```python
from build123d import *

# Parameters (mm, degrees)
ESQUISSE2_R          = 3.5
BOSS_EXTRU_1_DEPTH   = 3.5
D_GAGEMENT_M31_D     = 3.4
D_GAGEMENT_M31_DEPTH = 3.5


with BuildPart() as part:
    # Esquisse1 → Révolution1 (revolve)
    with BuildSketch(Plane.XY, mode=Mode.PRIVATE) as r_volution1_sk:
        Polygon((0, 0), (-9.5, 0), (-9.5, 3.5), (-7.5, 3.5), (-6.95, 6), (-16.95, 6), (-16.95, 26), (-2.5, 26), (-2.5, 42), (0, 42), align=None)
    revolve(r_volution1_sk.sketch.rotate(Axis((0, 0, 0), (0, 1, 0)), 270), axis=Axis((0, 0, 0), (0, 1, 0)))

    # Esquisse2 → Boss.-Extru.1 (add)
    with BuildSketch(Plane(origin=(0, 0, 0), x_dir=(-1, 0, 0), z_dir=(0, -1, 0))):
        with Locations((6.717514421, -6.717514421)):
            Circle(ESQUISSE2_R)
        with Locations((-6.717514421, -6.717514421)):
            Circle(ESQUISSE2_R)
        with Locations((-6.717514421, 6.717514421)):
            Circle(ESQUISSE2_R)
        with Locations((6.717514421, 6.717514421)):
            Circle(ESQUISSE2_R)
    extrude(amount=-BOSS_EXTRU_1_DEPTH)

    # Dégagement M31
    with Locations(Plane(origin=(-6.717514421, 0, 6.717514421), x_dir=(0, 0, -1), z_dir=(0, -1, 0))):
        with Locations((0, 0), (0, 13.435028842), (13.435028842, 13.435028842), (13.435028842, 0)):
            Hole(D_GAGEMENT_M31_D / 2, depth=D_GAGEMENT_M31_DEPTH)


solid = part.part
```
Could you check a few things on this model? Use its own coordinates, in mm. A direction names the side the tool comes from. Coordinates: 2 decimals unless noted, no trailing zeros. Write each loop counter-clockwise with the first axis right and the second up, starting at its lowest first coordinate (ties: lowest second). Pieces come first, ordered by that corner, then holes. Notation, with made-up numbers: (5.25, -25.75) - (42.25, -25.75) arc R15 cw to (42.25, -18.75) - close; hole circle Ø1 at (81, 83). An arc over 180 degrees is marked (long way). Use a Markdown table: item, result.
Q1. I'm going to push flat-ended pins straight in: pin 1 Ø8 at (x, y) = (2, 23.5) entering from +Z; pin 2 Ø4 at (x, z) = (-6.72, 6.72) entering from +Y; pin 3 Ø1.5 at (x, y) = (-4, 21) entering from -Z; pin 4 Ø8 at (y, z) = (25, -12) entering from +X. Where does each tip first touch, or does it pass through?
Geometry check:
| item | result |
|---|---|
| pin 1 | stops at z = 16.95 |
| pin 2 | stops at y = 26 |
| pin 3 | stops at z = -16.64 |
| pin 4 | stops at x = 14.94 |
Q2. Imagine slicing it at B-B (z = 0). List the corners of the cut face in (x, y) for me.
Geometry check:
| item | result |
|---|---|
| outline | (-16.95, 6) - (-6.95, 6) - (-7.5, 3.5) - (-9.5, 3.5) - (-9.5, 0) - (9.5, 0) - (9.5, 3.5) - (7.5, 3.5) - (6.95, 6) - (16.95, 6) - (16.95, 26) - (2.5, 26) - (2.5, 42) - (-2.5, 42) - (-2.5, 26) - (-16.95, 26) - close |
Q3. Please list where these lines run through material, in increasing order: L1, parallel to Y at x = 9, z = -8.5; L2, parallel to Y at x = -9, z = -14; L3, parallel to Y at x = -5, z = -4.
Geometry check:
| item | result |
|---|---|
| L1 | y = 0 to 3.5, 6 to 26 |
| L2 | y = 6 to 26 |
| L3 | y = 0 to 26 |
Q4. Thinking about a two-plate mould opening in X: for faces 1 (the cylindrical face through (7.866, 1.774, -7.97)), 2 (the cylindrical face through (2.44, 34.11, 0.54)), 3 (the flat face through (0, 0, 0)), which applies, +X half, -X half, draft (parallel to the pull), parting line (faces both ways), or undercut?
Geometry check:
| item | result |
|---|---|
| face 1 | undercut |
| face 2 | parting line |
| face 3 | draft |
Q5. Imagine slicing it at C-C (y = 30). List the corners of the cut face in (x, z) for me.
Geometry check:
| item | result |
|---|---|
| outline | circle Ø5 at (0, 0) |
Q6. Imagine slicing it at A-A (x = 0). List the corners of the cut face in (y, z) for me, and give its area (3 significant figures).
Geometry check:
| item | result |
|---|---|
| outline | (0, -9.5) - (3.5, -9.5) - (3.5, -7.5) - (6, -6.95) - (6, -16.95) - (26, -16.95) - (26, -2.5) - (42, -2.5) - (42, 2.5) - (26, 2.5) - (26, 16.95) - (6, 16.95) - (6, 6.95) - (3.5, 7.5) - (3.5, 9.5) - (0, 9.5) - close |
| area | 861 mm2 |
Q7. Which directions (+Z, -Z, +X, -X, +Y, -Y) give clear straight access to the entire face, cutting with the end or side of a thin tool? Please do faces 4 (the cylindrical face through (-0.1, 1.8, 9.5)), 5 (the cylindrical face through (0.1, 1.8, -9.5)), 6 (the flat face through (-7, 3.5, 4)), 7 (the cylindrical face through (8.15, 1.77, 7.63)).
Geometry check:
| item | result |
|---|---|
| face 4 | +Z, -Y |
| face 5 | -Z, -Y |
| face 6 | none |
| face 7 | -Y |
